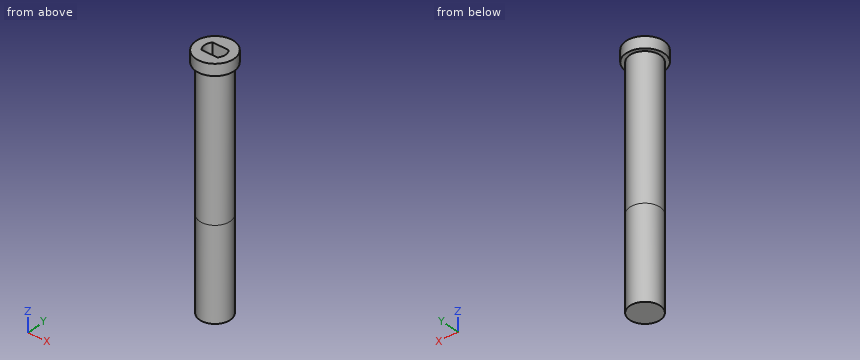
```python
from build123d import *

# Parameters (mm, degrees)
SKETCH1_R               = 4
BOSS_EXTRUDE1_DEPTH     = 40
SKETCH2_R               = 5
BOSS_EXTRUDE2_DEPTH     = 3
CUT_EXTRUDE1_DEPTH      = 43
CUT_EXTRUDE1_DEPTH_BACK = 3
SKETCH1_3_R             = 4
BOSS_EXTRUDE3_DEPTH     = 23
BOSS_EXTRUDE4_START     = 24
SKETCH3_R               = 4
BOSS_EXTRUDE4_DEPTH     = 24


with BuildPart() as part:
    # Sketch1 → Boss-Extrude1 (new body)
    with BuildSketch(Plane.XY):
        Circle(SKETCH1_R)
        with BuildLine():
            Line((-2.100590034, 1.75), (2.142050653, 1.75))
            ThreePointArc((2.142050653, 1.75), (2.766022596, 0), (2.142050653, -1.75))
            Line((2.142050653, -1.75), (-2.100590034, -1.75))
            ThreePointArc((-2.100590034, -1.75), (-2.733195007, 0), (-2.100590034, 1.75))
        make_face(mode=Mode.SUBTRACT)
    extrude(amount=BOSS_EXTRUDE1_DEPTH)

    # Sketch2 → Boss-Extrude2 (add)
    with BuildSketch(Plane.XY.offset(40)):
        Circle(SKETCH2_R)
    extrude(amount=-BOSS_EXTRUDE2_DEPTH)

    # Sketch1_2 → Cut-Extrude1 (cut, two sides: drawn at the far end of the back side and taken through both)
    with BuildSketch(Plane.XY.offset(-CUT_EXTRUDE1_DEPTH_BACK)):
        with BuildLine():
            ThreePointArc((-2.100590034, -1.75), (-2.733195007, 0), (-2.100590034, 1.75))
            Line((-2.100590034, 1.75), (2.142050653, 1.75))
            ThreePointArc((2.142050653, 1.75), (2.766022596, 0), (2.142050653, -1.75))
            Line((2.142050653, -1.75), (-2.100590034, -1.75))
        make_face()
    extrude(amount=CUT_EXTRUDE1_DEPTH + CUT_EXTRUDE1_DEPTH_BACK, mode=Mode.SUBTRACT)

    # Sketch1_3 → Boss-Extrude3 (add)
    with BuildSketch(Plane.XY):
        Circle(SKETCH1_3_R)
    extrude(amount=BOSS_EXTRUDE3_DEPTH)

    # Sketch3 → Boss-Extrude4 (add)
    with BuildSketch(Plane(origin=(0, 0, 0), x_dir=(-1, 0, 0), z_dir=(0, 0, -1)).offset(BOSS_EXTRUDE4_START)):
        Circle(SKETCH3_R)
    extrude(amount=-BOSS_EXTRUDE4_DEPTH)


solid = part.part
```
CAD build for the part. Positions are in the model's coordinates, mm. Give positions to 0.01 mm unless a question says otherwise; leave off trailing zeros. Order: outer loops, then holes, each group sorted by start corner. A loop starts at its lowest first (then second) coordinate and runs counter-clockwise, first axis right, second up. Notation, with made-up numbers: M -19,3 L -1,3 A17 ccw -1,18 Z; hole C 15,3 d4. An arc over 180 degrees is marked long. Put each result on its own line as item: value. Start each with the question number.
(1) Saw through at B-B, the plane y = 0. Write the cut outline in (x, z), then the cut area to 3 significant figures.
(2) Saw through at A-A, the plane z = 32. Write the cut outline in (x, y).
(3) Drill centre lines: line 1 along X through (y, z) = (-0.25, 34); line 2 along Z through (x, y) = (4.75, -0.25); line 3 along Y through (x, z) = (0, -2). Where is each one in solid material? Low to high.
(4) Saw through at D-D, the plane z = 16. Write the cut outline in (x, y), then the cut area to 3 significant figures.
(5) Saw through at C-C, the plane x = 0. Write the cut outline in (y, z).
(6) Flat gauge pins, fed straight in: pin 1 Ø6 at (x, y) = (-3, 3) entering from -Z; pin 2 Ø2 at (y, z) = (0, 7) entering from +X; pin 3 Ø1.3 at (x, z) = (0.5, 28) entering from -Y; pin 4 Ø2 at (x, z) = (-3, -4) entering from +Y. Where does each tip first touch, or does it go through?
Check result:
1. outline: M -5,37 L -4,37 L -4,-24 L 4,-24 L 4,37 L 5,37 L 5,40 L 2.77,40 L 2.77,23 L -2.73,23 L -2.73,40 L -5,40 Z
1. area: 425 mm2
2. outline: C 0,0 d8; hole M -2.1,-1.75 L 2.14,-1.75 A2.77 ccw 2.14,1.75 L -2.1,1.75 A2.74 ccw Z
3. line 1: x = -3.99 to -2.72, 2.75 to 3.99
3. line 2: z = 37 to 40
3. line 3: y = -4 to 4
4. outline: C 0,0 d8
4. area: 50.3 mm2
5. outline: M -5,37 L -4,37 L -4,-24 L 4,-24 L 4,37 L 5,37 L 5,40 L 1.75,40 L 1.75,23 L -1.75,23 L -1.75,40 L -5,40 Z
6. pin 1: stops at z = -24
6. pin 2: stops at x = 4
6. pin 3: stops at y = -4
6. pin 4: stops at y = 3.46
